Here's how the part is built. I have some questions about the finished solid (model axes, mm). Face numbers are marked on the shaded views. A direction names the side the tool comes from. Give positions to 0.01 mm unless a question says otherwise; leave off trailing zeros. Order: outer loops, then holes, each group sorted by start corner. A loop starts at its lowest first (then second) coordinate and runs counter-clockwise, first axis right, second up.
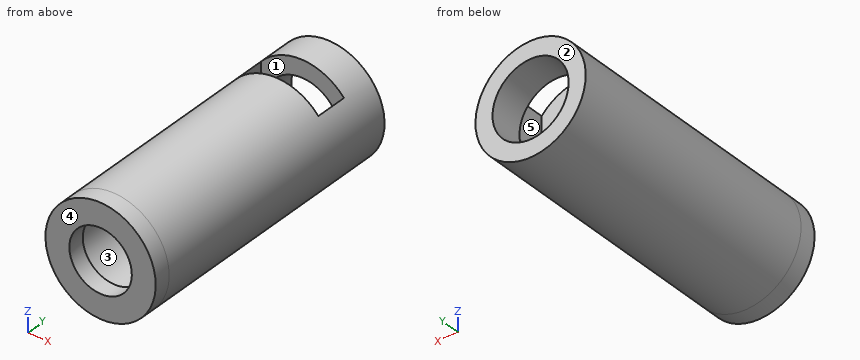
from build123d import *

# Parameters (mm, degrees)
SKETCH1_R           = 16.15
SKETCH1_R_2         = 11.15
BOSS_EXTRUDE1_DEPTH = 80
BOSS_EXTRUDE2_START = 5
SKETCH2_R           = 16.15
SKETCH2_R_2         = 9.15
BOSS_EXTRUDE2_DEPTH = 5
CUT_EXTRUDE1_DEPTH  = 9.5


with BuildPart() as part:
    # Sketch1 → Boss-Extrude1 (new body)
    with BuildSketch(Plane(origin=(0, 0, 0), x_dir=(1, 0, 0), z_dir=(0, 1, 0))):
        with Locations(Location((0, 0, 0), (0, 0, 270))):
            Circle(SKETCH1_R)
        with Locations(Location((0, 0, 0), (0, 0, 270))):
            Circle(SKETCH1_R_2, mode=Mode.SUBTRACT)
    extrude(amount=BOSS_EXTRUDE1_DEPTH)

    # Sketch2 → Boss-Extrude2 (add)
    with BuildSketch(Plane.XZ.offset(BOSS_EXTRUDE2_START)):
        with Locations(Location((0, 0, 0), (0, 0, 270))):
            Circle(SKETCH2_R)
        with Locations(Location((0, 0, 0), (0, 0, 270))):
            Circle(SKETCH2_R_2, mode=Mode.SUBTRACT)
    extrude(amount=-BOSS_EXTRUDE2_DEPTH)

    # Sketch4 → Cut-Extrude1 (cut)
    with BuildSketch(Plane(origin=(0, 70, 0), x_dir=(1, 0, 0), z_dir=(0, 1, 0))):
        with BuildLine():
            Line((-12.15, 0), (-12.15, -18.126783329))
            Line((-12.15, -18.126783329), (12.15, -18.126783329))
            Line((12.15, -18.126783329), (12.15, 0))
            ThreePointArc((12.15, 0), (0, 12.15), (-12.15, 0))
        make_face()
    extrude(amount=-CUT_EXTRUDE1_DEPTH, mode=Mode.SUBTRACT)


solid = part.part
Q1. If we section it at B-B on z = 5: List the corners of the cut face in (x, y) for me.
Filled sheet:
outline: (-15.36, -5) - (-7.66, -5) - (-7.66, 0) - (-9.97, 0) - (-9.97, 60.5) - (-12.15, 60.5) - (-12.15, 70) - (-9.97, 70) - (-9.97, 80) - (-15.36, 80) - close; (7.66, -5) - (15.36, -5) - (15.36, 80) - (9.97, 80) - (9.97, 70) - (12.15, 70) - (12.15, 60.5) - (9.97, 60.5) - (9.97, 0) - (7.66, 0) - close
Q2. Thinking about a two-plate mould opening in X: for the marked faces 1 and 2, which applies, released by +X, released by -X, zero draft, split by the parting line, or undercut?
Filled sheet:
face 1: undercut
face 2: zero draft
Q3. If we section it at A-A on x = 0: List the corners of the cut face in (y, z) for me.
Filled sheet:
outline: (-5, -16.15) - (80, -16.15) - (80, -11.15) - (70, -11.15) - (70, -12.15) - (60.5, -12.15) - (60.5, -11.15) - (0, -11.15) - (0, -9.15) - (-5, -9.15) - close; (-5, 9.15) - (0, 9.15) - (0, 11.15) - (60.5, 11.15) - (60.5, 16.15) - (-5, 16.15) - close; (70, 11.15) - (80, 11.15) - (80, 16.15) - (70, 16.15) - close
Q4. I'm going to push flat-ended pins straight in: P1, Ø3, axis at y = 39.5, z = -10, coming from the +X side; P2, Ø12, axis at x = -7, y = 32.5, coming from the -Z side; P3, Ø12, axis at x = 7.5, y = 54, coming from the +Z side; P4, Ø18, axis at x = 0, z = 0, coming from the -Y side. Where does each tip first touch, or does it pass through?
Filled sheet:
P1: stops at x = 13.73
P2: stops at z = -16.12
P3: stops at z = 16.08
P4: passes through
Q5. For the marked faces 3, 4 and 5, which set-ups out of +Z, -Z, +X, -X, +Y, -Y let a thin tool reach every point of the face, with its end or its side?
Filled sheet:
face 3: +Y
face 4: +Z, -Z, +X, -X, -Y
face 5: +Z
Q6. If we section it at C-C on y = 9: List the corners of the cut face in (x, z) for me.
Filled sheet:
outline: circle Ø32.3 at (0, 0); hole circle Ø22.3 at (0, 0)
Q7. I need wall thicknesses on L1, parallel to X at y = 38, z = 0; L2, parallel to Y at x = -5, z = 10.5. Which ranges of each line are inside material? Lowest first, please.
Filled sheet:
L1: x = -16.15 to -11.15, 11.15 to 16.15
L2: y = -5 to 60.5, 70 to 80
Q8. If we section it at D-D on x = -5: List the corners of the cut face in (y, z) for me, plus the area to 3 significant figures.
Filled sheet:
outline: (-5, -15.36) - (80, -15.36) - (80, -9.97) - (70, -9.97) - (70, -11.07) - (60.5, -11.07) - (60.5, -9.97) - (0, -9.97) - (0, -7.66) - (-5, -7.66) - close; (-5, 7.66) - (0, 7.66) - (0, 9.97) - (60.5, 9.97) - (60.5, 15.36) - (-5, 15.36) - close; (70, 9.97) - (80, 9.97) - (80, 15.36) - (70, 15.36) - close
area: 878 mm2
